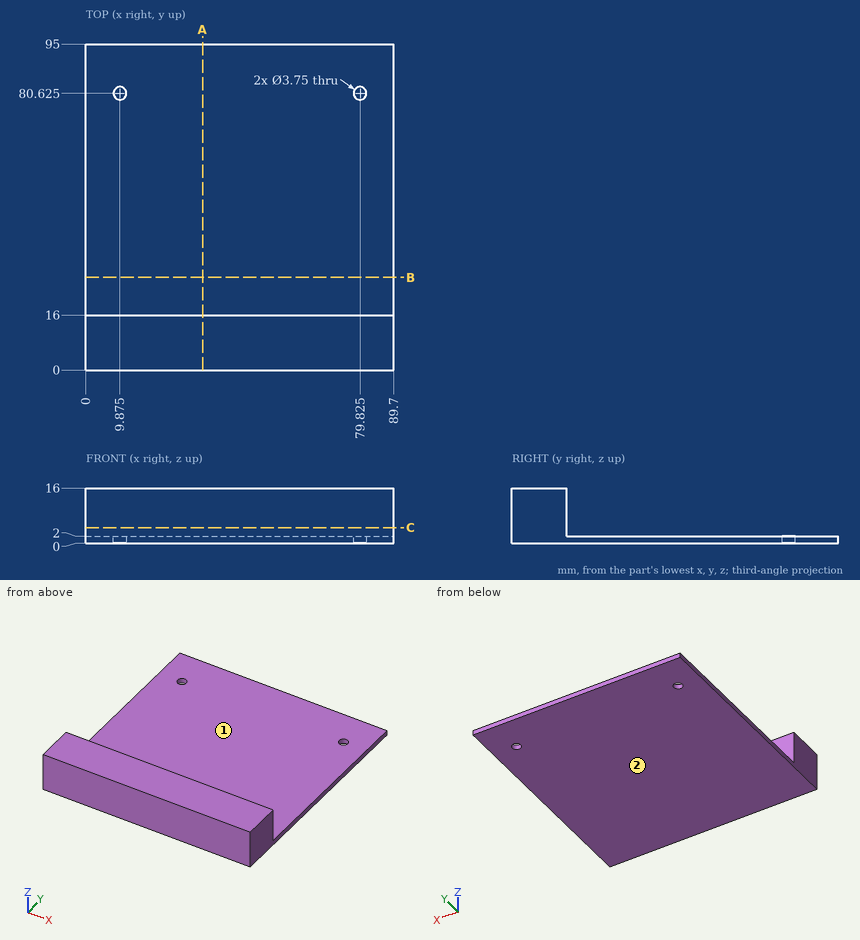
Geometry check sheet. Reference: drawing and pictorial views, mm from the part's lowest x, y, z. A direction names the side the tool comes from. Round coordinates to 2 decimals unless told otherwise and drop trailing zeros. Loops run counter-clockwise (first coordinate to the right, second up) from the corner with the lowest first, then second, coordinate; pieces in that order, holes last. Notation, with made-up numbers: (26.25, -39) - (70.25, -39) arc R23 cw to (70.25, -3) - close; hole circle Ø10 at (42.25, 8.5). An arc over 180 degrees is marked (long way). Answer in a Markdown table with one row per item. Add a question column.
Q1. Section check B-B on y = 27. Enter the section's corners in (x, z), plus the area to 3 significant figures.
Q2. Gauge pin test, flat ends, axial feed: pin 1 (3 mm diameter, centred on x = 64.5, y = 51.5, fed in from +Z); pin 2 (4 mm diameter, centred on x = 44, z = 12, fed in from +Y). Record the tip position at first contact, or that the pin passes through.
Q3. Section check C-C on z = 4.5. Enter the section's corners in (x, y), plus the area to 3 significant figures.
Q4. Section check A-A on x = 34. Enter the section's corners in (y, z).
Q5. Tool access check on the marked faces 1 and 2. Record the directions out of +Z, -Z, +X, -X, +Y, -Y that give a thin tool (end or side, any length) a straight path to the whole face; none if there is none.
Q6. Material ranges on line 1 (Y direction, x = 25.5, z = 11.5); line 2 (Z direction, x = 67.5, y = 54.5), recorded low to high.
Found:
| question | item | result |
|---|---|---|
| 1 | outline | (0, 0) - (89.7, 0) - (89.7, 2) - (0, 2) - close |
| 1 | area | 179 mm² |
| 2 | pin 1 | stops at z = 2 |
| 2 | pin 2 | stops at y = 16 |
| 3 | outline | (0, 0) - (89.7, 0) - (89.7, 16) - (0, 16) - close |
| 3 | area | 1,440 mm² |
| 4 | outline | (0, 0) - (95, 0) - (95, 2) - (16, 2) - (16, 16) - (0, 16) - close |
| 5 | face 1 | +Z, +X, -X, +Y |
| 5 | face 2 | -Z, +X, -X, +Y, -Y |
| 6 | line 1 | y = 0 to 16 |
| 6 | line 2 | z = 0 to 2 |
